For this review, take the finished solid that the model builds, in its own axes (mm). A direction names the side the tool comes from. Coordinates: 2 decimals unless noted, no trailing zeros. Order: outer loops, then holes, each group sorted by start corner. A loop starts at its lowest first (then second) coordinate and runs counter-clockwise, first axis right, second up. Notation, with made-up numbers: (86, 66) -> (115, 66) arc R12 ccw to (115, 83) -> close; hole circle Ø2 at (50, 57.25). An arc over 180 degrees is marked (long way). Return JSON: item names as keys, results as strings. Group by question number.
Item 1: Machinability: for faces 1 (the flat face through (21.406, -12.92, 54.65)), 2 (the flat face through (-21.406, 12.92, 54.65)), 3 (the flat face through (-10, -18, 80)), 4 (the flat face through (-12.92, -21.406, 54.65)), 5 (the flat face through (12.92, 21.406, 54.65)), which of the approach directions +Z, -Z, +X, -X, +Y, -Y give a long, thin tool a straight path to every point of the face, cutting with its end or side? Answer none if there is none.
Item 2: Take a section at C-C (z = 51). Write out the cut boundary in (x, y) (3 decimals).
Item 3: Insertion check: pin 1 (6 mm diameter, centred on y = -21, z = 110.5, fed in from -X); pin 2 (12 mm diameter, centred on x = -22, y = -5.5, fed in from +Z); pin 3 (3 mm diameter, centred on x = 3.5, z = 118, fed in from +Y); pin 4 (1.5 mm diameter, centred on x = -9, z = 107, fed in from -Y). Each pin has a flat end and moves straight along its axis. Give the tip position at first contact, or say it passes through.
Item 4: For line 1 along Y through (x, z) = (1, 24); line 2 along Z through (x, y) = (16, 30.5); line 3 along Z through (x, y) = (16, -20), list the stretches that pass through material, from the lowest coordinate up.
Item 5: Take a section at A-A (x = 20). Write out the cut boundary in (y, z), then the cut area to 3 significant figures.
Item 6: Take a section at B-B (y = 22). Write out the cut boundary in (x, z).
Item 7: Take a section at D-D (y = 2). Write out the cut boundary in (x, z), then the cut area to 3 significant figures.
```python
from build123d import *

# Parameters (mm, degrees)
F0_R     = 40
F1_DEPTH = 30
F3_DEPTH = 50


with BuildPart() as f1:
    # F0 (on Top) → F1 (new body)
    with BuildSketch(Plane.XY):
        Circle(F0_R)
    extrude(amount=F1_DEPTH)

    # F2 (on face) → F3 (join)
    with BuildSketch(Plane.XY.offset(30)):
        Polygon((34.199837, 8.964997), (-8.964997, 34.199837), (-34.199837, -8.964997), (8.964997, -34.199837), align=None)
    extrude(amount=F3_DEPTH)

    # F4 (on face) → F6 section 0
    with BuildSketch(Plane.XY.offset(80), mode=Mode.PRIVATE) as f6_s0:
        Polygon((-7.121267, 27.464645), (-27.375315, -7.028449), (7.117778, -27.282497), (27.371827, 7.210596), align=None)
    loft([f6_s0.sketch, Vertex(0, 0, 150.282912)])


solid = f1.part
```
Findings below:
{
 "1": {"face 1": "+Z, +X, -Y", "face 2": "+Z, -X, +Y", "face 3": "+Z", "face 4": "+Z, -X, -Y", "face 5": "+Z, +X, +Y"},
 "2": {"outline": "(-34.2, -8.965) -> (8.965, -34.2) -> (34.2, 8.965) -> (-8.965, 34.2) -> close"},
 "3": {"pin 1": "passes through", "pin 2": "stops at z = 108.81", "pin 3": "stops at y = 9.65", "pin 4": "stops at y = -9.45"},
 "4": {"line 1": "y = -39.99 to 39.99", "line 2": "z = 0 to 30", "line 3": "z = 0 to 80"},
 "5": {"outline": "(-34.64, 0) -> (34.64, 0) -> (34.64, 30) -> (17.27, 30) -> (17.27, 80) -> (11.54, 80) -> (5.27, 98.93) -> (-5.34, 80) -> (-15.32, 80) -> (-15.32, 30) -> (-34.64, 30) -> close", "area": "3,870 mm2"},
 "6": {"outline": "(-33.41, 0) -> (33.41, 0) -> (33.41, 30) -> (11.9, 30) -> (11.9, 80) -> (2.19, 80) -> (-5.7, 93.98) -> (-10.33, 80) -> (-16.1, 80) -> (-16.1, 30) -> (-33.41, 30) -> close"},
 "7": {"outline": "(-39.95, 0) -> (39.95, 0) -> (39.95, 30) -> (30.13, 30) -> (30.13, 80) -> (24.31, 80) -> (7.59, 130.79) -> (-0.52, 145.16) -> (-22.07, 80) -> (-27.79, 80) -> (-27.79, 30) -> (-39.95, 30) -> close", "area": "6,890 mm2"}
}
